from build123d import *

# Parameters (mm, degrees)
ESQUISSE1_R             = 7.5
ESQUISSE1_R_2           = 5
BOSS_EXTRU_1_DEPTH      = 2
ESQUISSE2_R             = 6
ESQUISSE2_R_2           = 5
BOSS_EXTRU_2_DEPTH      = 30
ESQUISSE3_R             = 6
ESQUISSE3_R_2           = 5
BOSS_EXTRU_3_DEPTH      = 20
ENL_V_MAT_EXTRU_1_DEPTH = 33
BOSS_EXTRU_4_DEPTH      = 3
ESQUISSE8_R             = 1.75
ENL_V_MAT_EXTRU_3_DEPTH = 16
ESQUISSE9_W             = 3
ESQUISSE9_H             = 5.8
ENL_V_MAT_EXTRU_4_DEPTH = 6


with BuildPart() as part:
    # Esquisse1 → Boss.-Extru.1 (new body)
    with BuildSketch(Plane.XY):
        Circle(ESQUISSE1_R)
        Circle(ESQUISSE1_R_2, mode=Mode.SUBTRACT)
    extrude(amount=BOSS_EXTRU_1_DEPTH)

    # Esquisse2 → Boss.-Extru.2 (add)
    with BuildSketch(Plane.XY.offset(2)):
        with Locations((0, 0.114284202)):
            Circle(ESQUISSE2_R)
        Circle(ESQUISSE2_R_2, mode=Mode.SUBTRACT)
    extrude(amount=BOSS_EXTRU_2_DEPTH)

    # Esquisse3 → Boss.-Extru.3 (add)
    with BuildSketch(Plane(origin=(0, 0, 0), x_dir=(-1, 0, 0), z_dir=(0, 0, -1))):
        Circle(ESQUISSE3_R)
        Circle(ESQUISSE3_R_2, mode=Mode.SUBTRACT)
    extrude(amount=BOSS_EXTRU_3_DEPTH)

    # Esquisse4 → Enlèv. mat.-Extru.1 (cut, through all)
    with BuildSketch(Plane(origin=(0, 0, 0), x_dir=(-1, 0, 0), z_dir=(0, 0, -1))):
        with BuildLine():
            Line((-6, 4.5), (-6, -4.5))
            ThreePointArc((-6, -4.5), (-7.5, 0), (-6, 4.5))
        make_face()
    extrude(amount=-ENL_V_MAT_EXTRU_1_DEPTH, mode=Mode.SUBTRACT)

    # Esquisse7 → Boss.-Extru.4 (add, symmetric)
    with BuildSketch(Plane(origin=(0, 0, -16), x_dir=(-1, 0, 0), z_dir=(0, 0, -1))):
        with BuildLine():
            Line((0, 6), (13, 6))
            Line((13, 6), (13, -6))
            Line((13, -6), (0, -6))
            ThreePointArc((0, -6), (6, 0), (0, 6))
        make_face()
    extrude(amount=BOSS_EXTRU_4_DEPTH, both=True)

    # Esquisse8 → Enlèv. mat.-Extru.3 (cut)
    with BuildSketch(Plane.ZY.offset(13)):
        with Locations((-16, 0)):
            Circle(ESQUISSE8_R)
    extrude(amount=-ENL_V_MAT_EXTRU_3_DEPTH, mode=Mode.SUBTRACT)

    # Esquisse9 → Enlèv. mat.-Extru.4 (cut)
    with BuildSketch(Plane(origin=(0, 0, -19), x_dir=(-1, 0, 0), z_dir=(0, 0, -1))):
        with Locations((9.5, 0)):
            Rectangle(ESQUISSE9_W, ESQUISSE9_H)
    extrude(amount=-ENL_V_MAT_EXTRU_4_DEPTH, mode=Mode.SUBTRACT)


solid = part.part
The listing builds one solid part. Answer for the finished solid, in the listing's coordinates (mm). A direction names the side the tool comes from. Round coordinates to 2 decimals unless told otherwise and drop trailing zeros. Loops run counter-clockwise (first coordinate to the right, second up) from the corner with the lowest first, then second, coordinate; pieces in that order, holes last. Notation, with made-up numbers: M -36,-30.75 L -30,-30.75 A25 cw -30,8.25 Z; hole C 49,-30 d4. An arc over 180 degrees is marked long. Write each question's results on one line, items separated by ' | '. Start each with the question number.
1) Straight lines are drawn through the part: probe 1 along Y at (x, z) = (0, -12.75); probe 2 along Y at (x, z) = (0, 16). For each, find the intervals that lie inside material, in ascending order.
2) Find section A-A on x = -4. Write down the section's boundary in (y, z).
3) Find section D-D on y = -1. Count the separate pieces of the cut face and the enclosed holes in it, plus the area to 3 significant figures.
4) Find section C-C on y = 4. Write down the section's boundary in (x, z).
5) Determine the mould class of faces 1 (the flat face through (6, 0, 1)), 2 (the cylindrical face through (-1.301, -5.743, 16.79)), 3 (the flat face through (-7, -6, -16)), 4 (the flat face through (-8, -1.3, -17.4)) for opening direction Y: pulls with the +Y half, pulls with the -Y half, needs draft (parallel to the pull), parting line crosses it, or undercut.
6) Which of the six approach directions +Z, -Z, +X, -X, +Y, -Y give full straight-line access (tool end or side, diameter ignored) to faces 5 (the flat face through (-6, 6, -16)), 6 (the cylindrical face through (-7.495, 0.262, 0.986)), 7 (the flat face through (-6, 2, 0)), 8 (the cylindrical face through (-12.014, 0.526, -14.331))?
7) Find section B-B on z = -16. Write down the section's boundary in (x, y), plus the area to 3 significant figures.
8) Each of these flat-tipped pins is pushed along its axis until it touches: pin 1 (5 mm diameter, centred on x = -8.5, y = -5.5, fed in from +Z); pin 2 (8 mm diameter, centred on x = -2, z = -10, fed in from +Y); pin 3 (1.7 mm diameter, centred on y = 1, z = -15, fed in from +X); pin 4 (6 mm diameter, centred on x = 0, y = 0, fed in from -Z). Where does it stop, or does it pass through?
Final values:
1) probe 1: -6 to -5, 5 to 6 | probe 2: -5.89 to -5, 5 to 6.11
2) outline: M -6.34,0 L -4.47,0 L -4.47,-13 L -6,-13 L -6,-19 L -4.47,-19 L -4.47,-20 L -3,-20 L -3,32 L -4.36,32 L -4.36,2 L -6.34,2 Z; M 3,-20 L 4.47,-20 L 4.47,-19 L 6,-19 L 6,-13 L 4.47,-13 L 4.47,0 L 6.34,0 L 6.34,2 L 4.59,2 L 4.59,32 L 3,32 Z
3) separate pieces: 5 | enclosed holes: 0 | area: 118 mm²
4) outline: M -13,-19 L -4.47,-19 L -4.47,-20 L -3,-20 L -3,32 L -4.57,32 L -4.57,2 L -6.34,2 L -6.34,0 L -4.47,0 L -4.47,-13 L -13,-13 Z; M 3,-20 L 4.47,-20 L 4.47,0 L 6,0 L 6,2 L 4.57,2 L 4.57,32 L 3,32 Z
5) face 1: needs draft | face 2: parting line crosses it | face 3: pulls with the -Y half | face 4: undercut
6) face 5: -Z, +X, -X, +Y | face 6: +Z | face 7: none | face 8: -X
7) outline: M -13,-6 L 0,-6 A6 ccw 0,6 L -13,6 L -13,1.75 L -11,1.75 L -11,2.9 L -8,2.9 L -8,1.75 L -4.68,1.75 A5 cw long -4.68,-1.75 L -8,-1.75 L -8,-2.9 L -11,-2.9 L -11,-1.75 L -13,-1.75 Z | area: 98.7 mm²
8) pin 1: z = -13 | pin 2: y = 6 | pin 3: x = 6 | pin 4: through
